For this review, take the finished solid that the model builds, in its own axes (mm). A direction names the side the tool comes from. Round coordinates to 2 decimals unless told otherwise and drop trailing zeros. Loops run counter-clockwise (first coordinate to the right, second up) from the corner with the lowest first, then second, coordinate; pieces in that order, holes last.
```python
from build123d import *

# Parameters (mm, degrees)
SKETCH1_W           = 7
SKETCH1_H           = 1.46
BOSS_EXTRUDE2_DEPTH = 2
SKETCH2_W           = 8
SKETCH2_H           = 8
BOSS_EXTRUDE3_DEPTH = 9.74993
BOSS_EXTRUDE4_DEPTH = 4.16
BOSS_EXTRUDE5_DEPTH = 8.64081
SKETCH6_R           = 1.5
BOSS_EXTRUDE7_DEPTH = 0.5
CIRPATTERN2_COUNT   = 4


with BuildPart() as part:
    # Sketch1 → Boss-Extrude2 (new body)
    with BuildSketch(Plane(origin=(0, 0, 0), x_dir=(1, 0, 0), z_dir=(0, 1, 0))):
        with BuildLine():
            Line((-67.759015818, -5.626850133), (-44.359015818, -5.626850133))
            ThreePointArc((-44.359015818, -5.626850133), (-42.237695475, -6.50552979), (-41.359015818, -8.626850133))
            Line((-41.359015818, -8.626850133), (-41.359015818, -10.626850133))
            ThreePointArc((-41.359015818, -10.626850133), (-42.237695475, -12.748170477), (-44.359015818, -13.626850133))
            Line((-44.359015818, -13.626850133), (-67.759015818, -13.626850133))
            ThreePointArc((-67.759015818, -13.626850133), (-69.880336162, -12.748170477), (-70.759015818, -10.626850133))
            Line((-70.759015818, -10.626850133), (-70.759015818, -8.626850133))
            ThreePointArc((-70.759015818, -8.626850133), (-69.880336162, -6.50552979), (-67.759015818, -5.626850133))
        make_face()
        with Locations((-64.559015818, -9.626850133)):
            Rectangle(SKETCH1_W, SKETCH1_H, mode=Mode.SUBTRACT)
        with Locations((-47.559015818, -9.626850133)):
            Rectangle(SKETCH1_W, SKETCH1_H, mode=Mode.SUBTRACT)
    extrude(amount=BOSS_EXTRUDE2_DEPTH)

    # Sketch2 → Boss-Extrude3 (add)
    with BuildSketch(Plane(origin=(0, 2, 0), x_dir=(1, 0, 0), z_dir=(0, 1, 0))):
        with Locations((-56.028566074, -9.626850133)):
            Rectangle(SKETCH2_W, SKETCH2_H)
    extrude(amount=BOSS_EXTRUDE3_DEPTH)

    # Sketch3 → Boss-Extrude4 (add)
    with BuildSketch(Plane(origin=(0, 11.74993, 0), x_dir=(1, 0, 0), z_dir=(0, 1, 0))):
        Polygon((-67.408566074, -8.126850133), (-57.528566074, -8.126850133), (-57.528566074, 1.753149867), (-54.528566074, 1.753149867), (-54.528566074, -8.126850133), (-44.648566074, -8.126850133), (-44.648566074, -11.126850133), (-54.528566074, -11.126850133), (-54.528566074, -21.006850133), (-57.528566074, -21.006850133), (-57.528566074, -11.126850133), (-67.408566074, -11.126850133), align=None)
    extrude(amount=BOSS_EXTRUDE4_DEPTH)

    # Sketch4 → Boss-Extrude5 (add)
    with BuildSketch(Plane(origin=(0, 11.74993, 0), x_dir=(1, 0, 0), z_dir=(0, 1, 0))):
        Polygon((-67.408566074, -8.126850133), (-69.723836074, -9.626850133), (-67.408566074, -11.126850133), align=None)
    boss_extrude5 = extrude(amount=BOSS_EXTRUDE5_DEPTH)

    # Sketch6 → Boss-Extrude7 (add)
    with BuildSketch(Plane(origin=(0, 0, 0), x_dir=(1, 0, 0), z_dir=(0, 1, 0))):
        with Locations((-56.028566074, -9.626850133)):
            Circle(SKETCH6_R)
    extrude(amount=BOSS_EXTRUDE7_DEPTH)

    # CirPattern2: Boss-Extrude5 ×4 about axis
    cirpattern2_axis = Axis((-56.028566074, 0, 9.626850133), (0, 1, 0))
    for i in range(1, CIRPATTERN2_COUNT):
        add(boss_extrude5.rotate(cirpattern2_axis, i * 360 / CIRPATTERN2_COUNT))


solid = part.part
```
(1) Add section C-C (x = -53.75). Give the boundary of the cut face in (y, z), plus the area to 3 significant figures.
(2) Add section B-B (x = -65.75). Give the boundary of the cut face in (y, z), plus the area to 3 significant figures.
(3) Add section D-D (z = 7.25). Give the boundary of the cut face in (x, y).
(4) For L1, parallel to Y at x = -61.25, z = 6.75; L2, parallel to Y at x = -54.75, z = 4.5; L3, parallel to X at y = 15, z = 20.5, list the stretches that pass through material, from the lowest coordinate up.
(5) Add section A-A (y = 18.75). Give the boundary of the cut face in (x, z), plus the area to 3 significant figures.
(6) Insertion check: pin 1 Ø2 at (x, z) = (-55.5, 19) entering from +Y; pin 2 Ø4.5 at (y, z) = (14, 4) entering from -X; pin 3 Ø5 at (y, z) = (5, 12.5) entering from +X; pin 4 Ø2 at (x, y) = (-49, 9) entering from +Z. Each pin has a flat end and moves straight along its axis. Give the tip position at first contact, or say it passes through.
(7) The part is to be moulded in two halves that separate along X. For faces 5 (the flat face through (-65, 1, 10.357)), 6 (the flat face through (-56, 15.91, 10)), 7 (the cylindrical face through (-69.904, 0.986, 6.529)), 8 (the flat face through (-56, 18, 21.007)), say which applies: pulls with the +X half, pulls with the -X half, needs draft (parallel to the pull), parting line crosses it, or undercut.
(8) For faces 1 (the flat face through (-56, 18, -1.753)), 2 (the flat face through (-63, 14, 8.127)), 3 (the flat face through (-57.529, 14, 16)), 4 (the flat face through (-50, 14, 8.127)), list the 3-axis set-ups (+Z, -Z, +X, -X, +Y, -Y) from which the entire face can be reached by the end or side of a thin tool; tool diameter is ignored.
Outcome:
1. outline: (0, 5.63) - (11.75, 5.63) - (11.75, 8.13) - (15.91, 8.13) - (15.91, 11.13) - (11.75, 11.13) - (11.75, 13.63) - (0, 13.63) - close
1. area: 106 mm2
2. outline: (0, 5.63) - (2, 5.63) - (2, 8.9) - (0, 8.9) - close; (0, 10.36) - (2, 10.36) - (2, 13.63) - (0, 13.63) - close; (11.75, 8.13) - (15.91, 8.13) - (15.91, 11.13) - (11.75, 11.13) - close
2. area: 25.6 mm2
3. outline: (-70.42, 0) - (-41.69, 0) - (-41.69, 2) - (-52.03, 2) - (-52.03, 11.75) - (-54.53, 11.75) - (-54.53, 15.91) - (-57.53, 15.91) - (-57.53, 11.75) - (-60.03, 11.75) - (-60.03, 2) - (-70.42, 2) - close
4. L1: y = 0 to 2
4. L2: y = 11.75 to 15.91
4. L3: x = -57.53 to -54.53
5. outline: (-69.72, 9.63) - (-67.41, 8.13) - (-67.41, 11.13) - close; (-57.53, -1.75) - (-56.03, -4.07) - (-54.53, -1.75) - close; (-57.53, 21.01) - (-54.53, 21.01) - (-56.03, 23.32) - close; (-44.65, 8.13) - (-42.33, 9.63) - (-44.65, 11.13) - close
5. area: 13.9 mm2
6. pin 1: stops at y = 15.91
6. pin 2: stops at x = -57.53
6. pin 3: stops at x = -52.03
6. pin 4: passes through
7. face 5: undercut
7. face 6: undercut
7. face 7: pulls with the -X half
7. face 8: needs draft
8. face 1: +X, -X, +Y
8. face 2: -Z, -X, +Y
8. face 3: +Z, -X, +Y
8. face 4: -Z, +X, +Y
